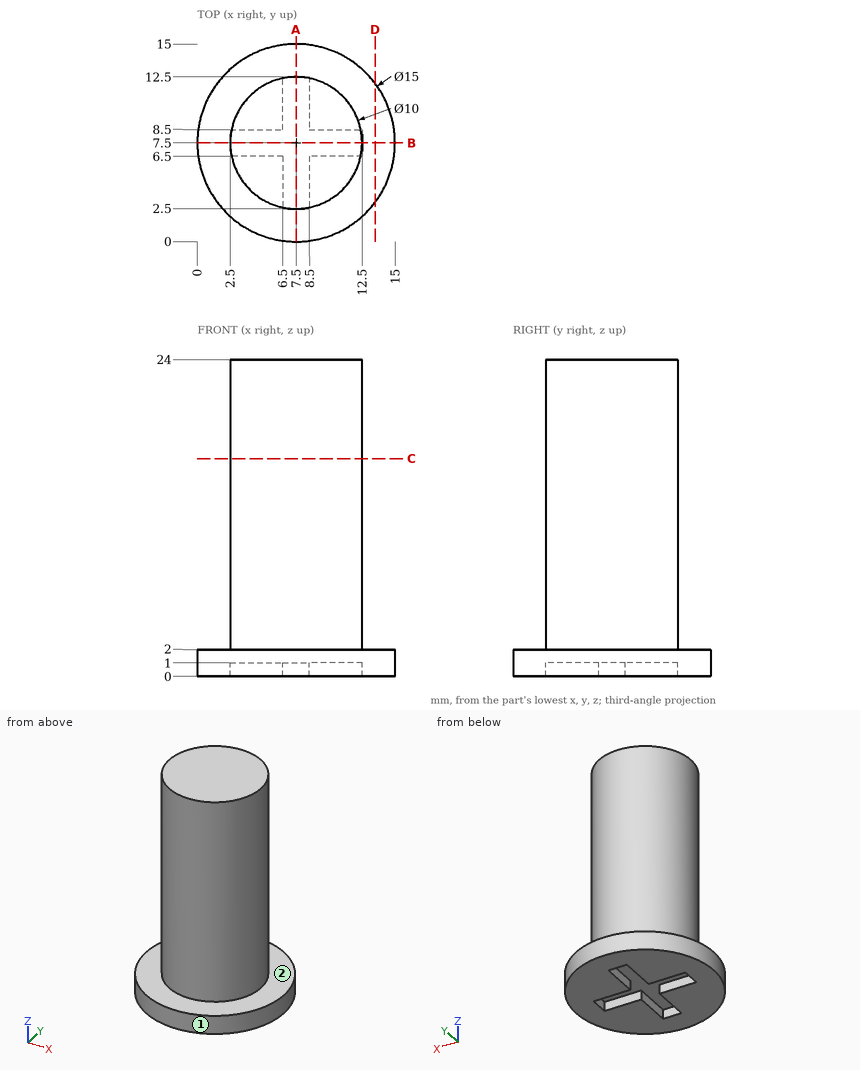
Job drawing, mm, ordinate dimensions from the low corner. One solid piece. A direction names the side the tool comes from. Coordinates: 2 decimals unless noted, no trailing zeros. Loops run counter-clockwise (first coordinate to the right, second up) from the corner with the lowest first, then second, coordinate; pieces in that order, holes last. Notation, with made-up numbers: (-23, -13) - (9, -13) arc R27 cw to (9, 15) - close; hole circle Ø6 at (-1, 2.5). An arc over 180 degrees is marked (long way). Answer as a JSON object with one key per item and string values. Group by question number.
(1) Cut at D-D (x = 13.5). Give the cut face in (y, z).
(2) Probe line 1 along Z through (x, y) = (13.75, 8.25); line 2 along Z through (x, y) = (7.25, 8); line 3 along X through (y, z) = (13.5, 1.75). List the from-to ranges inside material, lowest first.
(3) Tool access for the marked faces 1 and 2: list every direction of +Z, -Z, +X, -X, +Y, -Y with a clear straight run to the whole face (end or side of a thin tool).
(4) Cut at A-A (x = 7.5). Give the cut face in (y, z), then the cut area to 3 significant figures.
(5) Flat gauge pins, fed straight in: pin 1 (4 mm diameter, centred on y = 11, z = 11.5, fed in from -X); pin 2 (4 mm diameter, centred on x = 3, z = 20.5, fed in from -Y); pin 3 (1.1 mm diameter, centred on y = 9.5, z = 0.5, fed in from -X). Where does each tip first touch, or does it go through?
(6) Cut at C-C (z = 16.5). Give the cut face in (x, y), then the cut area to 3 significant figures.
Geometry says:
{
 "1": {"outline": "(3, 0) - (12, 0) - (12, 2) - (3, 2) - close"},
 "2": {"line 1": "z = 0 to 2", "line 2": "z = 1 to 24", "line 3": "x = 3 to 12"},
 "3": {"face 1": "+Z, -Z", "face 2": "+Z"},
 "4": {"outline": "(0, 0) - (2.5, 0) - (2.5, 1) - (12.5, 1) - (12.5, 0) - (15, 0) - (15, 2) - (12.5, 2) - (12.5, 24) - (2.5, 24) - (2.5, 2) - (0, 2) - close", "area": "240 mm^2"},
 "5": {"pin 1": "stops at x = 2.73", "pin 2": "stops at y = 3.17", "pin 3": "stops at x = 0.14"},
 "6": {"outline": "circle Ø10 at (7.5, 7.5)", "area": "78.5 mm^2"}
}
